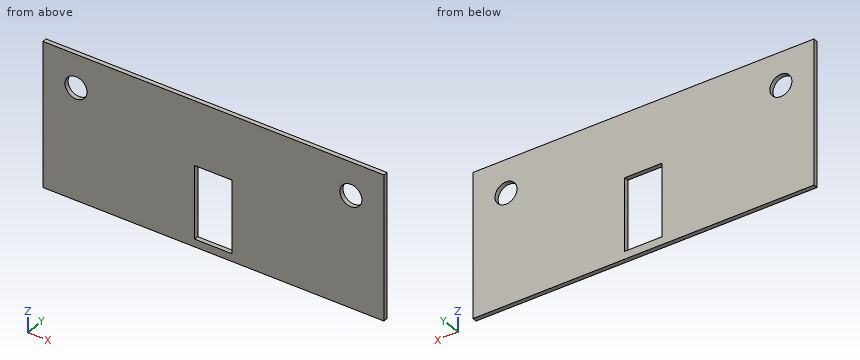
from build123d import *

# Parameters (mm, degrees)
SKETCH_1_W          = 154.889723794
SKETCH_1_H          = 65.431275614
SKETCH_1_W_2        = 17
SKETCH_1_H_2        = 32.940924084
EXTRUDE_1_DEPTH     = 2
SKETCH_2_R          = 5
CUT_EXTRUDE_2_DEPTH = 90.609556274


with BuildPart() as part:
    # Эскиз1 → Вытянуть1 (new body)
    with BuildSketch(Plane(origin=(0, 0, 0), x_dir=(1, 0, 0), z_dir=(0, 1, 0))):
        with Locations((0, -12.319525582)):
            Rectangle(SKETCH_1_W, SKETCH_1_H)
        with Locations((0, 0.417277171)):
            Rectangle(SKETCH_1_W_2, SKETCH_1_H_2, mode=Mode.SUBTRACT)
    extrude(amount=EXTRUDE_1_DEPTH)

    # Эскиз2 → Вытянуть2 (cut, through all)
    with BuildSketch(Plane(origin=(0, 2, 0), x_dir=(1, 0, 0), z_dir=(0, 1, 0))):
        with Locations(Location((-62.444861897, -30.035163389, 0), (0, 0, 270))):
            Circle(SKETCH_2_R)
        with Locations(Location((62.444861897, -30.035163389, 0), (0, 0, 90))):
            Circle(SKETCH_2_R)
    extrude(amount=-CUT_EXTRUDE_2_DEPTH, mode=Mode.SUBTRACT)


solid = part.part
Geometry check sheet. Reference: the model listing, model coordinates, mm. Give positions to 0.01 mm unless a question says otherwise; leave off trailing zeros. Order: outer loops, then holes, each group sorted by start corner. A loop starts at its lowest first (then second) coordinate and runs counter-clockwise, first axis right, second up. Notation, with made-up numbers: (-38.5, 28.25) - (-4.5, 28.25) arc R30 cw to (-4.5, 54.25) - close; hole circle Ø4 at (-2.75, 41.5). An arc over 180 degrees is marked (long way). Answer as a JSON object with one key per item and string values.
(1) Cross-section at B-B (z = -13). Record the cut outline in (x, y).
Report:
{"outline": "(-77.44, 0) - (-8.5, 0) - (-8.5, 2) - (-77.44, 2) - close; (8.5, 0) - (77.44, 0) - (77.44, 2) - (8.5, 2) - close"}
(2) Material ranges on line 1 (X direction, y = 0.3, z = 14); line 2 (Z direction, x = -63, y = 1.45); line 3 (X direction, y = 1.65, z = 27), recorded low to high.
Report:
{"line 1": "-77.44 to -8.5, 8.5 to 77.44", "line 2": "-20.4 to 25.07, 35 to 45.04", "line 3": "-77.44 to -66.42, -58.47 to 58.47, 66.42 to 77.44"}
(3) Cross-section at A-A (x = -2.5). Record the cut outline in (y, z), then the cut area to 3 significant figures.
Report:
{"outline": "(0, -20.4) - (2, -20.4) - (2, -16.89) - (0, -16.89) - close; (0, 16.05) - (2, 16.05) - (2, 45.04) - (0, 45.04) - close", "area": "65.0 mm^2"}
(4) Cross-section at D-D (y = 0.7). Record the cut outline in (x, z).
Report:
{"outline": "(-77.44, -20.4) - (77.44, -20.4) - (77.44, 45.04) - (-77.44, 45.04) - close; hole circle Ø10 at (-62.44, 30.04); hole (-8.5, -16.89) - (8.5, -16.89) - (8.5, 16.05) - (-8.5, 16.05) - close; hole circle Ø10 at (62.44, 30.04)"}
(5) Cross-section at C-C (z = 30). Record the cut outline in (x, y).
Report:
{"outline": "(-77.44, 0) - (-67.44, 0) - (-67.44, 2) - (-77.44, 2) - close; (-57.44, 0) - (57.44, 0) - (57.44, 2) - (-57.44, 2) - close; (67.44, 0) - (77.44, 0) - (77.44, 2) - (67.44, 2) - close"}
